The drawing under review shows one solid part. Ordinate dimensions are in mm from its lowest x, y, z. A direction names the side the tool comes from. Coordinates: 2 decimals unless noted, no trailing zeros. Order: outer loops, then holes, each group sorted by start corner. A loop starts at its lowest first (then second) coordinate and runs counter-clockwise, first axis right, second up. Notation, with made-up numbers: (14, 70.25) -> (59, 70.25) arc R15 ccw to (59, 82.25) -> close; hole circle Ø6 at (17, 34). An arc over 180 degrees is marked (long way). Use one line per item in the form item = value.
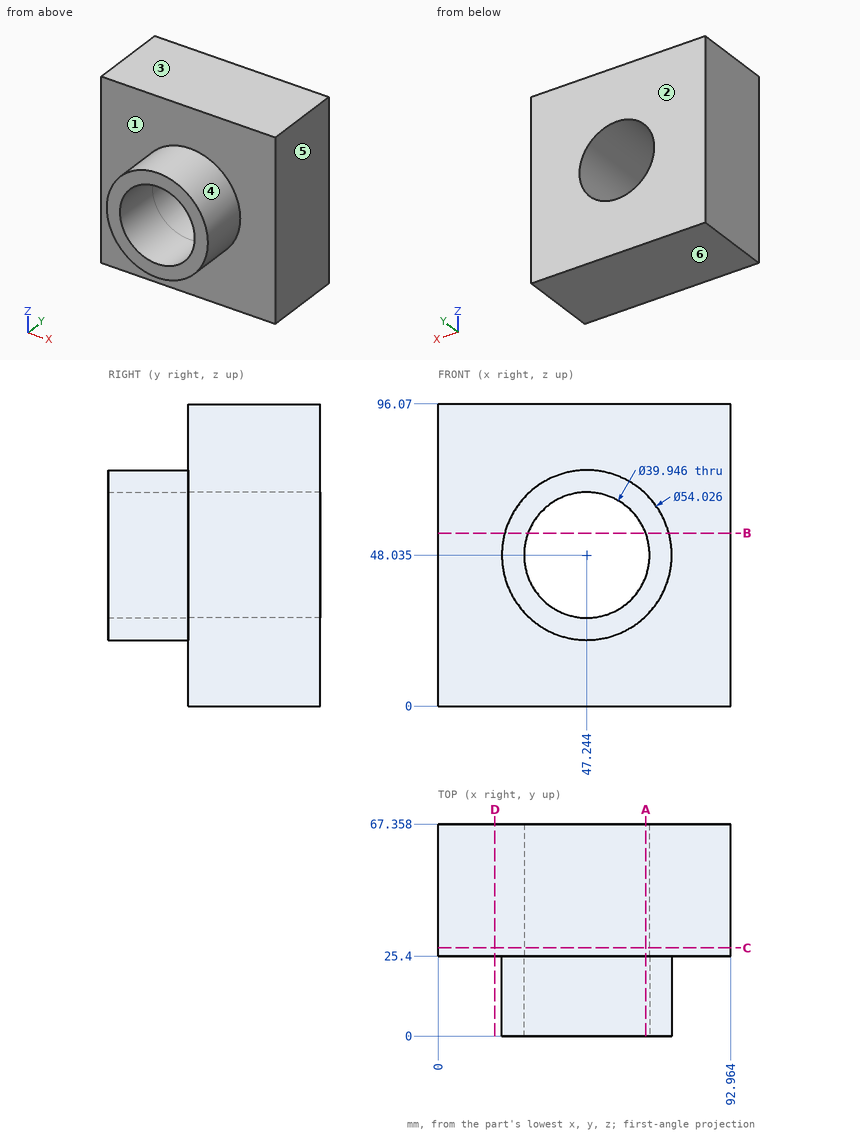
Item 1: We need section B-B (z = 55). Write out the cut boundary in (x, y) (1 decimal).
Results found:
outline = (0, 25.4) -> (21.1, 25.4) -> (21.1, 0) -> (28.5, 0) -> (28.5, 67.4) -> (0, 67.4) -> close; (66, 0) -> (73.3, 0) -> (73.3, 25.4) -> (93, 25.4) -> (93, 67.4) -> (66, 67.4) -> close
Item 2: Clearance check with a flat-ended pin moving along its axis: pin 1 (5 mm diameter, centred on x = 51, z = 81, fed in from -Y). State where the tip first meets the part, or that it passes through.
Results found:
pin_1 = 25.4
Item 3: To check wall thickness, follow L1, parallel to Y at x = 83, z = 12; L2, parallel to X at y = 44, z = 39.5; L3, parallel to X at y = 17.5, z = 46 (1 decimal). State the ranges of each line that lie inside material, in increasing order. Write a range as from..to.
Results found:
L1 = 25.4..67.36
L2 = 0..29.19, 65.3..92.96
L3 = 20.3..27.4, 67.1..74.2
Item 4: We need section A-A (x = 66). Write out the cut boundary in (y, z) (1 decimal), plus the area to 3 significant figures.
Results found:
outline = (0, 28.6) -> (25.4, 28.6) -> (25.4, 0) -> (67.4, 0) -> (67.4, 41.2) -> (0, 41.2) -> close; (0, 54.9) -> (67.4, 54.9) -> (67.4, 96.1) -> (25.4, 96.1) -> (25.4, 67.5) -> (0, 67.5) -> close
area = 4,090 mm²
Item 5: We need section C-C (y = 28). Write out the cut boundary in (x, z) (1 decimal).
Results found:
outline = (0, 0) -> (93, 0) -> (93, 96.1) -> (0, 96.1) -> close; hole circle Ø39.9 at (47.2, 48)
Item 6: Draft analysis for pull direction Z (two halves, no side actions). For the marked faces 3, 4, 5 and 6, state which applies: released by +Z, released by -Z, zero draft, split by the parting line, or undercut.
Results found:
face_3 = released by +Z
face_4 = split by the parting line
face_5 = zero draft
face_6 = released by -Z
Item 7: We need section D-D (x = 18). Write out the cut boundary in (y, z), plus the area to 3 significant figures.
Results found:
outline = (25.4, 0) -> (67.36, 0) -> (67.36, 96.07) -> (25.4, 96.07) -> close
area = 4,030 mm²
Item 8: Tool access review of the marked faces 1 and 2: name each direction out of +Z, -Z, +X, -X, +Y, -Y from which nothing blocks a thin tool from reaching the whole face with its end or side.
Results found:
face_1 = -Y
face_2 = +Z, -Z, +X, -X, +Y
